CAD build for the part. Positions are in the model's coordinates, mm. A direction names the side the tool comes from. Coordinates: 2 decimals unless noted, no trailing zeros. Write each loop counter-clockwise with the first axis right and the second up, starting at its lowest first coordinate (ties: lowest second). Pieces come first, ordered by that corner, then holes. Notation, with made-up numbers: M -12,84 L 16,84 A21 ccw 16,120 Z; hole C 84.25,16.5 d9. An arc over 180 degrees is marked long. Put each result on its own line as item: value. Start each with the question number.
```python
from build123d import *

# Parameters (mm, degrees)
PAD_DEPTH   = 8
FILLET_R    = 6
FILLET001_R = 23


with BuildPart() as part:
    # Sketch → Pad (new body)
    with BuildSketch(Plane.XY):
        Polygon((-8, 6), (0, 6), (0, 12), (400, 12), (420, 6), (420, -6), (400, -12), (0, -12), (0, -6), (-8, -6), align=None)
    extrude(amount=PAD_DEPTH)

    # Fillet
    fillet_edges = [part.edges().sort_by_distance(p)[0] for p in [
        (420, -6, 4),
        (420, 6, 4),
    ]]
    fillet(fillet_edges, radius=FILLET_R)

    # Fillet001
    fillet001_edges = [part.edges().sort_by_distance(p)[0] for p in [
        (400, 12, 4),
        (400, -12, 4),
    ]]
    fillet(fillet001_edges, radius=FILLET001_R)


solid = part.part
```
(1) Which spindle directions (+Z, -Z, +X, -X, +Y, -Y) get a long thin tool onto all of the face, cutting with end or side? Do faces 1 (the face through (-4, -6, 4)), 2 (the face through (400.01, -11.75, 4.06)), 3 (the face through (-4, 6, 4)). Say none if no direction does.
(2) Drill centre lines: line 1 (X direction, y = -2.5, z = 5); line 2 (X direction, y = -2, z = 5); line 3 (Y direction, x = 399, z = 1.5). Where is each one in solid material? Low to high. Write a range as [from, to].
(3) Drop flat-ended pins along their axis: pin 1 (3 mm diameter, centred on x = 149.5, y = 5.5, fed in from -Z); pin 2 (1.8 mm diameter, centred on y = 9.5, z = 4.5, fed in from -X); pin 3 (2.5 mm diameter, centred on x = -4.5, z = 2.5, fed in from +Y). Give the stop position or say it passes through.
(4) Slice it at A-A, the plane z = 2.5. Write the cut outline in (x, y).
Result set:
1. face 1: +Z, -Z, -X, -Y
1. face 2: +Z, -Z, +X, -Y
1. face 3: +Z, -Z, -X, +Y
2. line 1: x = [-8, 419.92]
2. line 2: x = [-8, 419.98]
2. line 3: y = [-11.88, 11.88]
3. pin 1: stops at z = 0
3. pin 2: stops at x = 0
3. pin 3: stops at y = 6
4. outline: M -8,-6 L 0,-6 L 0,-12 L 396.62,-12 A23 ccw 403.23,-11.03 L 415.72,-7.28 A6 ccw 420,-1.54 L 420,1.54 A6 ccw 415.72,7.28 L 403.23,11.03 A23 ccw 396.62,12 L 0,12 L 0,6 L -8,6 Z
